```python
from build123d import *

# Parameters (mm, degrees)
ESQUISSE1_R        = 1
BOSS_EXTRU_1_DEPTH = 8
CHANFREIN1_SIZE    = 8


with BuildPart() as part:
    # Esquisse1 → Boss.-Extru.1 (new body)
    with BuildSketch(Plane.XY):
        with BuildLine():
            Line((5.879855223, 335.703540816), (5.879855223, 368.656410216))
            Line((5.879855223, 368.656410216), (-3.120144777, 368.656410216))
            Line((-3.120144777, 368.656410216), (-3.120144777, 521.656410212))
            Line((-3.120144777, 521.656410212), (13.879855223, 521.656410212))
            Line((13.879855223, 521.656410212), (13.879855223, 571.582220472))
            Line((13.879855223, 571.582220472), (8.001175566, 571.582220472))
            ThreePointArc((8.001175566, 571.582220472), (5.879855223, 571.582220472), (5.879855223, 573.703540816))
            Line((5.879855223, 573.703540816), (5.879855223, 596.798102411))
            Line((5.879855223, 596.798102411), (5.879855223, 606.656410212))
            Line((5.879855223, 606.656410212), (-84.120144777, 606.656410212))
            Line((-84.120144777, 606.656410212), (-84.120144777, 596.798102411))
            Line((-84.120144777, 596.798102411), (-84.120144777, -23.417779528))
            Line((-84.120144777, -23.417779528), (5.879855223, -23.417779528))
            Line((5.879855223, -23.417779528), (5.879855223, 54.460900128))
            ThreePointArc((5.879855223, 54.460900128), (5.879855223, 56.582220472), (8.001175566, 56.582220472))
            Line((8.001175566, 56.582220472), (13.879855223, 56.582220472))
            Line((13.879855223, 56.582220472), (13.879855223, 106.582220472))
            Line((13.879855223, 106.582220472), (8.001175566, 106.582220472))
            ThreePointArc((8.001175566, 106.582220472), (5.879855223, 106.582220472), (5.879855223, 108.703540816))
            Line((5.879855223, 108.703540816), (5.879855223, 166.119071534))
            Line((5.879855223, 166.119071534), (-4.120144777, 166.119071534))
            ThreePointArc((-4.120144777, 166.119071534), (-19.120144777, 181.119071534), (-4.120144777, 196.119071534))
            Line((-4.120144777, 196.119071534), (5.879855223, 196.119071534))
            Line((5.879855223, 196.119071534), (5.879855223, 225.04536941))
            Line((5.879855223, 225.04536941), (-4.120144777, 225.04536941))
            ThreePointArc((-4.120144777, 225.04536941), (-19.120144777, 240.04536941), (-4.120144777, 255.04536941))
            Line((-4.120144777, 255.04536941), (5.879855223, 255.04536941))
            Line((5.879855223, 255.04536941), (5.879855223, 281.460900128))
            ThreePointArc((5.879855223, 281.460900128), (5.879855223, 283.582220472), (8.001175566, 283.582220472))
            Line((8.001175566, 283.582220472), (13.879855223, 283.582220472))
            Line((13.879855223, 283.582220472), (13.879855223, 333.582220472))
            Line((13.879855223, 333.582220472), (8.001175566, 333.582220472))
            ThreePointArc((8.001175566, 333.582220472), (5.879855223, 333.582220472), (5.879855223, 335.703540816))
        make_face()
        with Locations((-60.550144777, 496.30133456)):
            Circle(ESQUISSE1_R, mode=Mode.SUBTRACT)
        with Locations((-36.550144777, 496.30133456)):
            Circle(ESQUISSE1_R, mode=Mode.SUBTRACT)
        with Locations((-60.550144777, 472.30133456)):
            Circle(ESQUISSE1_R, mode=Mode.SUBTRACT)
        with Locations((-36.550144777, 472.30133456)):
            Circle(ESQUISSE1_R, mode=Mode.SUBTRACT)
        with Locations((-60.593593351, 321.744120307)):
            Circle(ESQUISSE1_R, mode=Mode.SUBTRACT)
        with Locations((-18.595445866, 321.995534365)):
            Circle(ESQUISSE1_R, mode=Mode.SUBTRACT)
        with Locations((-18.28416987, 269.997586055)):
            Circle(ESQUISSE1_R, mode=Mode.SUBTRACT)
        with Locations((-60.282317355, 269.746171996)):
            Circle(ESQUISSE1_R, mode=Mode.SUBTRACT)
        with BuildLine():
            Line((-61.998824434, 214.582220472), (-16.241465121, 214.582220472))
            ThreePointArc((-16.241465121, 214.582220472), (-14.120144777, 214.582220472), (-14.120144777, 212.460900128))
            Line((-14.120144777, 212.460900128), (-14.120144777, 208.703540816))
            ThreePointArc((-14.120144777, 208.703540816), (-14.120144777, 206.582220472), (-16.241465121, 206.582220472))
            Line((-16.241465121, 206.582220472), (-61.998824434, 206.582220472))
            ThreePointArc((-61.998824434, 206.582220472), (-64.120144777, 206.582220472), (-64.120144777, 208.703540816))
            Line((-64.120144777, 208.703540816), (-64.120144777, 212.460900128))
            ThreePointArc((-64.120144777, 212.460900128), (-64.120144777, 214.582220472), (-61.998824434, 214.582220472))
        make_face(mode=Mode.SUBTRACT)
    extrude(amount=BOSS_EXTRU_1_DEPTH)

    # Chanfrein1
    chanfrein1_edges = [part.edges().sort_by_distance(p)[0] for p in [
        (-39.120144777, 606.656410212, 8),
    ]]
    chamfer(chanfrein1_edges, length=CHANFREIN1_SIZE - 0.0001)  # a hair under: the kernel refuses the full size


solid = part.part
```
Check sheet for the modelled part. Datum: model origin and axes. Units: mm. Round coordinates to 2 decimals unless told otherwise and drop trailing zeros. Order: outer loops, then holes, each group sorted by start corner. A loop starts at its lowest first (then second) coordinate and runs counter-clockwise, first axis right, second up. Notation, with made-up numbers: (-5.5, 3) -> (46.5, 3) arc R25 cw to (46.5, 31) -> close; hole circle Ø6 at (-28.5, 43.25). An arc over 180 degrees is marked (long way). One line per item, written item: value. Start each with the question number.
Q1. Mould release check, pull along Y, two halves, no side actions. Record for faces 1 (the face through (-19.117, 180.789, 3.944)), 2 (the face through (-36, 292, 8)): pulls with the +Y half, pulls with the -Y half, needs draft (parallel to the pull), parting line crosses it, or undercut.
Q2. Cross-section at B-B (y = 374). Record the boundary of the cut face in (x, z).
Q3. Cross-section at D-D (y = 33.5). Record the boundary of the cut face in (x, z), and give its area (3 significant figures).
Q4. Cross-section at C-C (z = 1.5). Give the number of separate pieces and of enclosed holes in the cut face, and give its area (3 significant figures).
Q5. Gauge pin test, flat ends, axial feed: pin 1 Ø1.8 at (x, y) = (-60.55, 472.3) entering from +Z; pin 2 Ø4 at (y, z) = (-2, 5) entering from +X; pin 3 Ø1.5 at (x, z) = (-4, 6.5) entering from +Y; pin 4 Ø2.5 at (y, z) = (441.5, 3.5) entering from +X. Record the tip position at first contact, or that the pin passes through.
Q6. Thickness scan on line 1 (Y direction, x = 6, z = 4.5); line 2 (Y direction, x = -17, z = 4.5); line 3 (X direction, y = 216, z = 1.5). Record the ranges inside material, lowest first.
Completed:
1. face 1: undercut
1. face 2: needs draft
2. outline: (-84.12, 0) -> (-3.12, 0) -> (-3.12, 8) -> (-84.12, 8) -> close
3. outline: (-84.12, 0) -> (5.88, 0) -> (5.88, 8) -> (-84.12, 8) -> close
3. area: 720 mm²
4. separate pieces: 1
4. enclosed holes: 9
4. area: 54,700 mm²
5. pin 1: passes through
5. pin 2: stops at x = 5.88
5. pin 3: stops at y = 600.91
5. pin 4: stops at x = -3.12
6. line 1: y = 56.69 to 106.47, 283.69 to 333.47, 521.66 to 571.47
6. line 2: y = -23.42 to 173.43, 188.81 to 206.58, 214.58 to 232.36, 247.73 to 602.16
6. line 3: x = -84.12 to 5.88
